from build123d import *

# Parameters (mm, degrees)
SKETCH1_W           = 29
SKETCH1_H           = 15
BOSS_EXTRUDE1_DEPTH = 15
SKETCH2_R           = 5.8
BOSS_EXTRUDE2_DEPTH = 20
SKETCH3_R           = 2.5
CUT_EXTRUDE1_DEPTH  = 8


with BuildPart() as part:
    # Sketch1 → Boss-Extrude1 (new body)
    with BuildSketch(Plane.XY):
        Rectangle(SKETCH1_W, SKETCH1_H)
    extrude(amount=BOSS_EXTRUDE1_DEPTH)

    # Sketch2 → Boss-Extrude2 (add)
    with BuildSketch(Plane(origin=(0, 7.5, 0), x_dir=(1, 0, 0), z_dir=(0, 1, 0))):
        with Locations((0, -7.5)):
            Circle(SKETCH2_R)
    extrude(amount=BOSS_EXTRUDE2_DEPTH)

    # Sketch3 → Cut-Extrude1 (cut)
    with BuildSketch(Plane(origin=(0, 0, 0), x_dir=(-1, 0, 0), z_dir=(0, 0, -1))):
        Circle(SKETCH3_R)
    extrude(amount=-CUT_EXTRUDE1_DEPTH, mode=Mode.SUBTRACT)


solid = part.part
For this review, take the finished solid that the model builds, in its own axes (mm). Round coordinates to 2 decimals unless told otherwise and drop trailing zeros. Order: outer loops, then holes, each group sorted by start corner. A loop starts at its lowest first (then second) coordinate and runs counter-clockwise, first axis right, second up. Notation, with made-up numbers: (-34.5, 8) -> (-12.5, 8) arc R21 ccw to (-12.5, 18) -> close; hole circle Ø9 at (-19, -8). An arc over 180 degrees is marked (long way). Write item = value, one per line. Start each with the question number.
1) Take a section at A-A on z = 7.5. State the section outline as (x, y) points.
2) Take a section at C-C on x = 0. State the section outline as (y, z) points, plus the area to 3 significant figures.
3) Insertion check: pin 1 (6 mm diameter, centred on y = 16, z = 9.5, fed in from +X); pin 2 (1.5 mm diameter, centred on x = 1.5, y = 17, fed in from -Z); pin 3 (8 mm diameter, centred on y = 12.5, z = 11.5, fed in from -X). Each pin has a flat end and moves straight along its axis. Give the tip position at first contact, or say it passes through.
4) The part is to be moulded in two halves that separate along X. For faces 1 (the face through (-0.76, 17.36, 1.75)), 2 (the face through (0.54, -2.44, 3.94)), 3 (the face through (-14.5, 0, 7)), 4 (the face through (0, 0, 8)), say which applies: +X half, -X half, draft (parallel to the pull), parting line (faces both ways), or undercut.
5) Take a section at B-B on y = -2. State the section outline as (x, z) points, plus the area to 3 significant figures.
6) To check wall thickness, follow line 1 (Y direction, x = 0, z = 6.25); line 2 (Y direction, x = -10.25, z = 7.25); line 3 (X direction, y = -2, z = 6.5). State the ranges of each line that lie inside material, in increasing order. Write a range as from..to.
7) Take a section at D-D on z = 11.5. State the section outline as (x, y) points.
Verdict:
q1.outline = (-14.5, -7.5) -> (14.5, -7.5) -> (14.5, 7.5) -> (5.8, 7.5) -> (5.8, 27.5) -> (-5.8, 27.5) -> (-5.8, 7.5) -> (-14.5, 7.5) -> close; hole circle Ø5 at (0, 0)
q2.outline = (-7.5, 0) -> (-2.5, 0) -> (-2.5, 8) -> (2.5, 8) -> (2.5, 0) -> (7.5, 0) -> (7.5, 1.7) -> (27.5, 1.7) -> (27.5, 13.3) -> (7.5, 13.3) -> (7.5, 15) -> (-7.5, 15) -> close
q2.area = 417 mm2
q3.pin_1 = 5.8
q3.pin_2 = 1.75
q3.pin_3 = -5.8
q4.face_1 = parting line
q4.face_2 = undercut
q4.face_3 = -X half
q4.face_4 = undercut
q5.outline = (-14.5, 0) -> (-1.5, 0) -> (-1.5, 8) -> (1.5, 8) -> (1.5, 0) -> (14.5, 0) -> (14.5, 15) -> (-14.5, 15) -> close
q5.area = 411 mm2
q6.line_1 = -7.5..-2.5, 2.5..27.5
q6.line_2 = -7.5..7.5
q6.line_3 = -14.5..-1.5, 1.5..14.5
q7.outline = (-14.5, -7.5) -> (14.5, -7.5) -> (14.5, 7.5) -> (4.2, 7.5) -> (4.2, 27.5) -> (-4.2, 27.5) -> (-4.2, 7.5) -> (-14.5, 7.5) -> close
